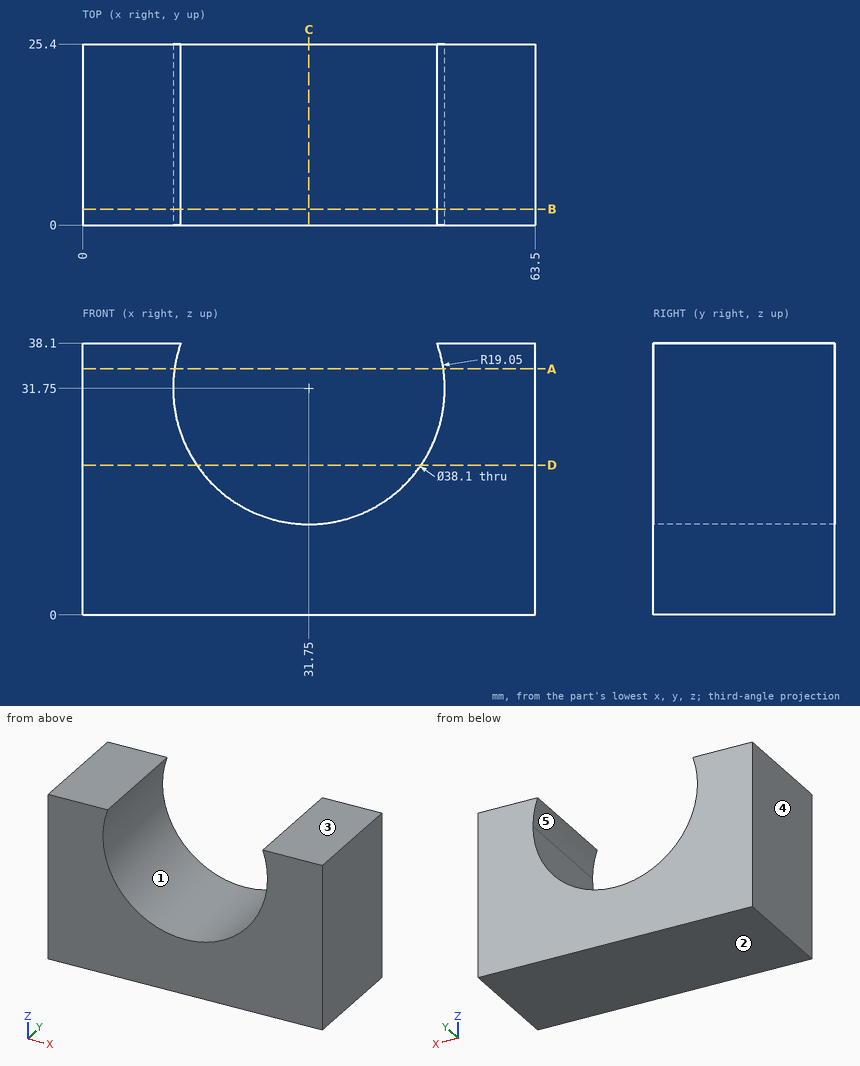
Design review of the part shown in the three views and the two pictorial views. Dimensions are in mm from the part's minimum x, y and z. A direction names the side the tool comes from. Round coordinates to 2 decimals unless told otherwise and drop trailing zeros. Write each loop counter-clockwise with the first axis right and the second up, starting at its lowest first coordinate (ties: lowest second). Pieces come first, ordered by that corner, then holes. Notation, with made-up numbers: (-3, -15) - (36, -15) arc R18 ccw to (36, 2) - close; hole circle Ø6 at (-24.75, -36). An arc over 180 degrees is marked (long way). Write item = value, one per line. Start each with the question number.
1. Draft analysis for pull direction Z (two halves, no side actions). For the marked faces 1, 2 and 3, state which applies: released by +Z, released by -Z, zero draft, split by the parting line, or undercut.
2. Wall thickness on L1, parallel to X at y = 10.5, z = 31.75; L2, parallel to Z at x = 31.75, y = 9.5; L3, parallel to X at y = 15.75, z = 15: over which ranges is each line inside the solid? List them lowest first.
3. Consider section D-D on z = 21. State the section outline as (x, y) points.
4. Consider section A-A on z = 34.5. State the section outline as (x, y) points.
5. For the marked faces 4 and 5, list the 3-axis set-ups (+Z, -Z, +X, -X, +Y, -Y) from which the entire face can be reached by the end or side of a thin tool; tool diameter is ignored.
6. Consider section B-B on y = 2.25. State the section outline as (x, z) points, plus the area to 3 significant figures.
7. Consider section C-C on x = 31.75. State the section outline as (y, z) points.
8. For pin 1 Ø12 at (x, y) = (28, 21.5) entering from -Z, flat-tipped, find the tip position at first contact; note if it passes through.
Evaluation:
q1.face_1 = undercut
q1.face_2 = released by -Z
q1.face_3 = released by +Z
q2.L1 = 0 to 12.7, 50.8 to 63.5
q2.L2 = 0 to 12.7
q2.L3 = 0 to 22.68, 40.82 to 63.5
q3.outline = (0, 0) - (16.02, 0) - (16.02, 25.4) - (0, 25.4) - close; (47.48, 0) - (63.5, 0) - (63.5, 25.4) - (47.48, 25.4) - close
q4.outline = (0, 0) - (12.9, 0) - (12.9, 25.4) - (0, 25.4) - close; (50.6, 0) - (63.5, 0) - (63.5, 25.4) - (50.6, 25.4) - close
q5.face_4 = +Z, -Z, -X, +Y, -Y
q5.face_5 = +Y, -Y
q6.outline = (0, 0) - (63.5, 0) - (63.5, 38.1) - (49.71, 38.1) arc R19.05 cw to (50.8, 31.75) arc R19.05 cw (long way) to (13.79, 38.1) - (0, 38.1) - close
q6.area = 1,610 mm2
q7.outline = (0, 0) - (25.4, 0) - (25.4, 12.7) - (0, 12.7) - close
q8.pin_1 = 0
